Design review of the part shown in the three views and the two pictorial views. Dimensions are in mm from the part's minimum x, y and z. Round coordinates to 2 decimals unless told otherwise and drop trailing zeros. Order: outer loops, then holes, each group sorted by start corner. A loop starts at its lowest first (then second) coordinate and runs counter-clockwise, first axis right, second up. Notation, with made-up numbers: (36.5, 28) - (46.5, 28) arc R28 ccw to (46.5, 67) - close; hole circle Ø1 at (84.5, -19.75). An arc over 180 degrees is marked (long way). One line per question, with ' | ' between items. Start each with the question number.
Item 1: For L1, parallel to X at y = 150, z = 3.5 (1 decimal); L2, parallel to X at y = 152, z = 1.25 (1 decimal), list the stretches that pass through material, from the lowest coordinate up. Write a range as [from, to].
Item 2: Insertion check: pin 1 Ø3 at (x, y) = (127.06, 105.07) entering from +Z. The pin has a flat end and moves straight along its axis. Give the tip position at first contact, or say it passes through.
Item 3: Add section B-B on y = 30. State the section outline as (x, z) points, and give its area (3 significant figures).
Item 4: Add section A-A on x = 7. State the section outline as (y, z) points.
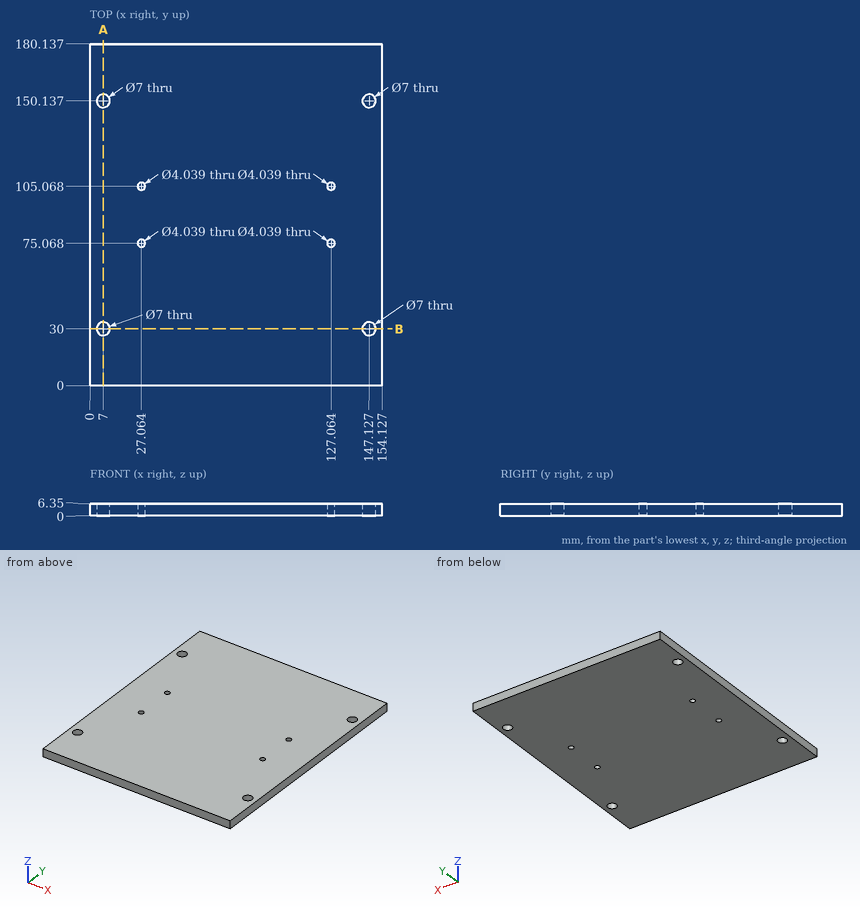
Determined:
1) L1: [0, 3.5], [10.5, 143.6], [150.6, 154.1] | L2: [0, 4], [10, 144.2], [150.1, 154.1]
2) pin 1: through
3) outline: (0, 0) - (3.5, 0) - (3.5, 6.35) - (0, 6.35) - close; (10.5, 0) - (143.63, 0) - (143.63, 6.35) - (10.5, 6.35) - close; (150.63, 0) - (154.13, 0) - (154.13, 6.35) - (150.63, 6.35) - close | area: 890 mm2
4) outline: (0, 0) - (26.5, 0) - (26.5, 6.35) - (0, 6.35) - close; (33.5, 0) - (146.64, 0) - (146.64, 6.35) - (33.5, 6.35) - close; (153.64, 0) - (180.14, 0) - (180.14, 6.35) - (153.64, 6.35) - close
